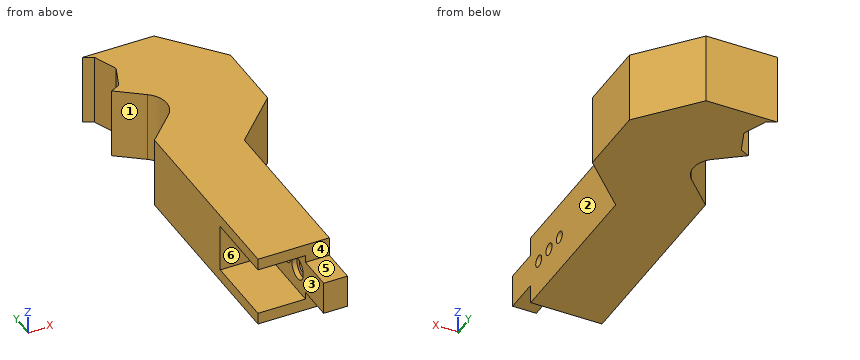
Autodesk Inventor part; units mm, degrees
ref_plane "YZ Plane" through (0, 0, 0) normal (1, 0, 0) x (0, 1, 0)
ref_plane "XZ Plane" through (0, 0, 0) normal (0, 1, 0) x (-1, 0, 0)
ref_plane "XY Plane" through (0, 0, 0) normal (0, 0, 1) x (1, 0, 0)
sketch "Sketch1" plane through (0, 0, 0) normal (0, 0, 1) x (1, 0, 0)
  line L0 (0, 0) -> (25, 0)
  line L1 (25, 0) -> (25, 40)
  line L2 (25, 40) -> (0, 40)
  line L3 (0, 40) -> (0, 0)
  dimension "d1" = 25
  dimension "d2" = 40
  dimension "d3" = 25
extrude "Extrusion1" add sketch "Sketch1" against normal blind 30
sketch "Sketch2" plane through (25, 0, 0) normal (1, 0, 0) x (0, 0, -1)
  line L0 (0, 0) -> (30, 0)
  circle A0 centre (15, 6.56) radius 2.46
extrude "Extrusion2" cut sketch "Sketch2" against normal blind 30
sketch "Sketch3" plane through (0, 0, 0) normal (-1, 0, 0) x (0, 0, 1)
  line L0 (0, 0) -> (-30, 0)
  line L1 (-25.05, 0) -> (-4.95, 0)
  line L2 (-4.95, 0) -> (-4.95, 33.12)
  line L3 (-4.95, 33.12) -> (-25.05, 33.12)
  line L4 (-25.05, 33.12) -> (-25.05, 0)
  dimension "d11" = 20.1
extrude "Extrusion3" cut sketch "Sketch3" against normal blind 20
sketch "Sketch4" plane through (0, 0, 0) normal (0, -1, 0) x (1, 0, 0)
  line L0 (20, -4.95) -> (20, -25.05)
  line L1 (20, -15) -> (25, -15)
  line L2 (25, 0) -> (25, -30)
  line L3 (20, -8.025) -> (25, -8.025)
  line L4 (25, -8.025) -> (25, -21.975)
  line L5 (25, -21.975) -> (20, -21.975)
  line L6 (20, -21.975) -> (20, -8.025)
  line L7 (20, -8.025) -> (25, -21.975) construction
  line L8 (25, -8.025) -> (20, -21.975) construction
  line L9 (25, -12.54) -> (25, -17.46)
  point P0 (0, 0)
  point P1 (22.5, -15)
  dimension "d14" = 13.95
extrude "Extrusion4" add sketch "Sketch4" along normal blind 15
sketch "Sketch5" plane through (20, 0, 0) normal (-1, 0, 0) x (0, 0, 1)
  circle A0 centre (-15, 6.56) radius 2.46
  circle A1 centre (-15, 6.56) radius 4.7025
  circle A2 centre (-15, 6.56) radius 2.46
  circle A3 centre (-15, 6.56) radius 2.46
  point P0 (0, 0)
  dimension "d17" = 9.405
extrude "Extrusion5" cut sketch "Sketch5" against normal blind 2.1
sketch "Sketch6" plane through (25, 0, 0) normal (1, 0, 0) x (0, 0, -1)
  circle A0 centre (15, 6.56) radius 4.7025
  line L0 (15, 6.56) -> (15, 23.56)
  circle A1 centre (15, 23.56) radius 2.46
  point P0 (0, 0)
  dimension "d20" = 17
  dimension "d21" = 4.92
extrude "Extrusion6" cut sketch "Sketch6" against normal blind 10 contours A1
sketch "Sketch7" plane through (20, 0, 0) normal (-1, 0, 0) x (0, 0, 1)
  circle A0 centre (-15, 23.56) radius 2.46
  circle A1 centre (-15, 23.56) radius 4.7025
  point P0 (0, 0)
  dimension "d24" = 9.405
extrude "Extrusion7" cut sketch "Sketch7" against normal blind 2.1
sketch "Sketch9" plane through (25, 0, 0) normal (1, 0, 0) x (0, 0, -1)
  circle A0 centre (15, 6.56) radius 2.46
  circle A1 centre (15, 6.56) radius 2.46
  circle A2 centre (15, 23.56) radius 2.46
  circle A3 centre (15, 23.56) radius 2.46
  line L0 (30, 40) -> (30, 0)
  line L1 (30, 0) -> (30, 40)
  line L2 (30, 40) -> (0, 40)
  line L3 (0, 40) -> (0, 0)
  line L4 (0, 0) -> (8.025, 0)
  line L5 (21.975, 0) -> (21.975, -15)
  line L6 (21.975, -15) -> (8.025, -15)
  line L7 (8.025, -15) -> (8.025, 0)
  line L8 (0, 0) -> (8.025, 0)
  line L9 (21.975, 0) -> (30, 0)
extrude "Extrusion8" add sketch "Sketch9" along normal blind 5
sketch "Sketch10" plane through (0, 40, 0) normal (0, 1, 0) x (1, 0, 0)
  line L0 (0, 30) -> (30, 30)
  line L1 (30, 0) -> (0, 0)
  line L2 (0, 30) -> (30, 30)
  line L3 (30, 30) -> (30, 0)
  line L4 (30, 0) -> (0, 0)
  line L5 (0, 0) -> (0, 30)
extrude "Extrusion9" add sketch "Sketch10" along normal blind 30
sketch "Sketch12" plane through (30, 0, 0) normal (1, 0, 0) x (0, 0, -1)
  circle A0 centre (15, 6.56) radius 2.46
  line L0 (15, 6.56) -> (15, 15.06)
  circle A1 centre (15, 15.06) radius 2.525
  point P0 (0, 0)
  dimension "d31" = 8.5
  dimension "d33" = 5.05
extrude "Extrusion10" cut sketch "Sketch12" against normal blind 30 contours A1
sketch "Sketch15" plane through (0, 0, -25.05) normal (-1, 0, 0) x (0, 0, 1)
  line L0 (0, 33.12) -> (20.1, 33.12)
  line L1 (20.1, 33.12) -> (20.1, 0)
  line L2 (0, 33.12) -> (20.1, 33.12)
  line L3 (20.1, 33.12) -> (20.1, 31.1)
  line L4 (20.1, 31.1) -> (0, 31.1)
  line L5 (0, 31.1) -> (0, 33.12)
  point P0 (25.05, 0)
  dimension "d57" = 2.02
extrude "Extrusion13" add sketch "Sketch15" against normal blind 20
sketch "Sketch17" plane through (0, 0, 0) normal (0, 0, 1) x (1, 0, 0)
  line L0 (0, 70) -> (30, 70)
  line L1 (30, 70) -> (50.0622, 90.0622)
  line L2 (30, 70) -> (80, 70) construction
  line L3 (11.9522, 97.2454) -> (0, 85.2932)
  line L4 (0, 70) -> (0, 85.2932)
  line L5 (0, 70) -> (0, 0)
  line L6 (0, 70) -> (30, 70)
  line L7 (10.923, 112.2849) -> (0, 120.567)
  line L8 (50.0622, 105.3553) -> (50.0622, 120.567)
  line L9 (50.0622, 105.3553) -> (50.0622, 90.0622)
  arc A0 (11.9522, 97.2454) -> (10.923, 112.2849) centre (4.8811, 104.3165) ccw
  line L10 (0, 144.567) -> (30, 144.567)
  line L11 (30, 144.567) -> (50.0622, 120.567)
  line L12 (4, 142.567) -> (0, 144.567)
  line L13 (4, 122.567) -> (0, 120.567)
  line L14 (4, 122.567) -> (8, 132.567)
  line L15 (8, 132.567) -> (4, 142.567)
  dimension "d61" = 45
  dimension "d62" = 32.0271
  dimension "d72" = 10
extrude "Extrusion14" add sketch "Sketch17" against normal blind 30
properties part number "rec_c_20mm_x_30mm"
Source: CAD feature listing. Evaluate the final solid. Frame: model axes, mm. Face numbers are marked on the shaded views. A direction names the side the tool comes from. Coordinates: 2 decimals unless noted, no trailing zeros. Write each loop counter-clockwise with the first axis right and the second up, starting at its lowest first coordinate (ties: lowest second). Pieces come first, ordered by that corner, then holes. Notation, with made-up numbers: M 29,-34 L 46,-34 A5 ccw 46,-28 Z; hole C 0,58.5 d9. An arc over 180 degrees is marked long. Answer as a JSON object with one key per item and string values.
1. Cut plane B-B on z = -3. Output: boundary loops of the cut face in (x, y).
Evaluation:
{"outline": "M 0,0 L 30,0 L 30,70 L 50.06,90.06 L 50.06,120.57 L 30,144.57 L 0,144.57 L 4,142.57 L 8,132.57 L 4,122.57 L 0,120.57 L 10.92,112.28 A10 cw 11.95,97.25 L 0,85.29 Z"}
2. Access query for the marked faces 1, 2 and 3. Directions: +Z, -Z, +X, -X, +Y, -Y. A direction counts if a zero-diameter tool reaches every point of the face in a straight line with its end or side. Return the directions, or none.
Evaluation:
{"face 1": "+Z, -Z, -X", "face 2": "+Z, -Z, +X, -Y", "face 3": "-X, -Y"}
3. Cut plane A-A on y = 6.56. Output: boundary loops of the cut face in (x, z), plus the area to 3 significant figures.
Evaluation:
{"outline": "M 0,-30 L 30,-30 L 30,-17.46 L 22.1,-17.46 L 22.1,-19.7 L 20,-19.7 L 20,-25.05 L 0,-25.05 Z; M 0,-4.95 L 20,-4.95 L 20,-10.3 L 22.1,-10.3 L 22.1,-12.54 L 30,-12.54 L 30,0 L 0,0 Z", "area": "439 mm^2"}
4. Draft query along Z for the marked faces 4, 5 and 6. Return one class per face: released by +Z, released by -Z, zero draft, split by the parting line, or undercut.
Evaluation:
{"face 4": "zero draft", "face 5": "released by +Z", "face 6": "undercut"}
5. Cut plane C-C on z = -15. State how many separate pieces and enclosed holes the cut face has, plus the area to 3 significant figures.
Evaluation:
{"separate pieces": "4", "enclosed holes": "0", "area": "4,300 mm^2"}
6. Ray query, L1, parallel to Y at x = 20.6, z = -15 (1 decimal); L2, parallel to Y at x = 23.75, z = -15 (3 decimals); L3, parallel to Z at x = 25, y = 6.56. Return the intervals inside material, ascending.
Evaluation:
{"L1": "-15 to 1.9, 11.3 to 12.5, 17.6 to 18.9, 28.3 to 144.6", "L2": "-15 to 4.1, 9.02 to 12.535, 17.585 to 21.1, 26.02 to 144.567", "L3": "-30 to -17.46, -12.54 to 0"}
7. Cut plane D-D on y = 74.5. Output: boundary loops of the cut face in (x, z).
Evaluation:
{"outline": "M 0,-30 L 34.5,-30 L 34.5,0 L 0,0 Z"}
8. Contact query for flat-ended pins moving along their axis: P1, Ø8, axis at y = 15.06, z = -15, coming from the -X side; P2, Ø5, axis at x = 26, y = -7.5, coming from the -Z side (3 decimals); P3, Ø4, axis at y = 19.5, z = -16.5, coming from the +X side; P4, Ø2, axis at x = 6, y = 93.5, coming from the +Z side. Output: stop coordinate, or through.
Evaluation:
{"P1": "x = 20", "P2": "z = -21.975", "P3": "x = 30", "P4": "through"}
